from build123d import *

# Parameters (mm, degrees)
SALIENTE_EXTRUIR1_OUTLINE_R = 1.5
SALIENTE_EXTRUIR1_DEPTH     = 3
S_LIDO_MOVER_COPIAR1_ANGLE  = 90


# Read off the part's stored shape, not the designer's step: Saliente-Extruir1
with BuildPart() as part:
    # Saliente-Extruir1 outline → Saliente-Extruir1 (new body)
    with BuildSketch(Plane.XY):
        with BuildLine():
            ThreePointArc((41771.487432324, -438.916733549), (41774.992492467, -434.200692189), (41770.014438295, -431.078918755))
            ThreePointArc((41770.014438295, -431.078918755), (41751.456517689, -433.102313751), (41733.174949659, -429.324111148))
            ThreePointArc((41733.174949659, -429.324111148), (41725.991842174, -431.730062122), (41726.889701646, -439.251995491))
            ThreePointArc((41726.889701646, -439.251995491), (41729.909074744, -445.69247761), (41727.882942515, -452.510924062))
            ThreePointArc((41727.882942515, -452.510924062), (41728.480324995, -457.995391332), (41733.987432324, -457.666733549))
            ThreePointArc((41733.987432324, -457.666733549), (41751.046402032, -444.909672965), (41771.487432324, -438.916733549))
        make_face()
        with Locations((41731.061313295, -454.939495491)):
            Circle(SALIENTE_EXTRUIR1_OUTLINE_R, mode=Mode.SUBTRACT)
        with BuildLine():
            Line((41738.411012413, -442.993278413), (41736.838856305, -443.404992792))
            ThreePointArc((41736.838856305, -443.404992792), (41735.982036246, -443.234989406), (41735.585699802, -442.456555601))
            ThreePointArc((41735.585699802, -442.456555601), (41735.69345686, -441.876829753), (41736.169165633, -441.52841218))
            Line((41736.169165633, -441.52841218), (41737.831630416, -441.093055392))
            ThreePointArc((41737.831630416, -441.093055392), (41738.100055673, -441.068468468), (41738.361410126, -441.134426674))
            Line((41738.361410126, -441.134426674), (41742.678233483, -443.044025097))
            Line((41742.678233483, -443.044025097), (41742.08574273, -437.173422628))
            ThreePointArc((41742.08574273, -437.173422628), (41742.914855043, -435.985031701), (41744.060436871, -436.872354922))
            Line((41744.060436871, -436.872354922), (41744.754133415, -443.73758562))
            ThreePointArc((41744.754133415, -443.73758562), (41744.580022463, -444.529990261), (41743.875600122, -444.932493559))
            Line((41743.875600122, -444.932493559), (41742.980225481, -445.023621226))
            Line((41742.980225481, -445.023621226), (41738.411012413, -442.993278413))
        make_face(mode=Mode.SUBTRACT)
        with Locations((41731.061313295, -434.939495491)):
            Circle(SALIENTE_EXTRUIR1_OUTLINE_R, mode=Mode.SUBTRACT)
        with Locations((41771.061313295, -434.939495491)):
            Circle(SALIENTE_EXTRUIR1_OUTLINE_R, mode=Mode.SUBTRACT)
    extrude(amount=SALIENTE_EXTRUIR1_DEPTH)


with BuildPart() as part_1:
    # Sólido-Mover/Copiar1: moved
    add(part.part.rotate(Axis((0, -443.939495491, 1.5), (-1, 0, 0)), S_LIDO_MOVER_COPIAR1_ANGLE))


solid = part_1.part
Here's how the part is built. I have some questions about the finished solid (model axes, mm). A direction names the side the tool comes from. Give positions to 0.01 mm unless a question says otherwise; leave off trailing zeros. Loops run counter-clockwise (first coordinate to the right, second up) from the corner with the lowest first, then second, coordinate; pieces in that order, holes last. Notation, with made-up numbers: (-18, 78) -> (19, 78) arc R37 ccw to (19, 114) -> close; hole circle Ø3 at (26, -0.75). An arc over 180 degrees is marked (long way). Answer as a JSON object with one key per item and string values. Group by question number.
Item 1: Thinking about a two-plate mould opening in Z: for faces 3 (the flat face through (41739, -442.439, -2)), 4 (the cylindrical face through (41750.779, -443.96, 2.605)), 5 (the cylindrical face through (41728.416, -443.96, 15.5)), which applies, pulls with the +Z half, pulls with the -Z half, needs draft (parallel to the pull), parting line crosses it, or undercut?
Item 2: Will these pins go through, and if not, where does the flat tip stop? pin 1 (2.5 mm diameter, centred on x = 41731.06, z = 12.5, fed in from +Y); pin 2 (4 mm diameter, centred on x = 41731.06, z = -7.5, fed in from -Y); pin 3 (1 mm diameter, centred on y = -445, z = 7.5, fed in from +X).
Item 3: Imagine slicing it at A-A on z = -7.5. Write out the boundary of the cut face in (x, y).
Item 4: I need wall thicknesses on L1, parallel to X at y = -443.25, z = -7.5; L2, parallel to Z at x = 41730.5, y = -444.05; L3, parallel to X at y = -443.6, z = -5. Which ranges of each line are inside material? Lowest first, please.
Item 5: On a 3-axis mill with a long thin cutter (end or side, diameter ignored), from which of +Z, -Z, +X, -X, +Y, -Y can I reach the whole of each face in a straight line? I mean faces 1 (the flat face through (41736.989, -443.96, -1.126)), 2 (the cylindrical face through (41751.719, -443.96, -9.325)). Say none if no direction works.
Item 6: Imagine slicing it at D-D on z = 12.5. Write out the boundary of the cut face in (x, y), then the cut area to 3 significant figures.
Item 7: Imagine slicing it at B-B on y = -443.7. Write out the boundary of the cut face in (x, z), then the cut area to 3 significant figures.
Item 8: Imagine slicing it at C-C on x = 41772. Write out the boundary of the cut face in (y, z).
Answer list:
{
 "1": {"face 3": "needs draft", "face 4": "pulls with the +Z half", "face 5": "undercut"},
 "2": {"pin 1": "passes through", "pin 2": "stops at y = -445.44", "pin 3": "stops at x = 41743.45"},
 "3": {"outline": "(41725.06, -445.44) -> (41729.56, -445.44) -> (41729.56, -442.44) -> (41725.06, -442.44) -> close; (41732.56, -445.44) -> (41769.56, -445.44) -> (41769.56, -442.44) -> (41732.56, -442.44) -> close; (41772.56, -445.44) -> (41775.06, -445.44) -> (41775.06, -442.44) -> (41772.56, -442.44) -> close"},
 "4": {"L1": "x = 41725.06 to 41729.56, 41732.56 to 41769.56, 41772.56 to 41775.06", "L2": "z = -13.47 to -8.89, -6.11 to 11.11, 13.89 to 16.46", "L3": "x = 41725.61 to 41742.11, 41744.12 to 41774.18"},
 "5": {"face 1": "+Y, -Y", "face 2": "-Z, +Y, -Y"},
 "6": {"outline": "(41727.06, -445.44) -> (41729.56, -445.44) -> (41729.56, -442.44) -> (41727.06, -442.44) -> close; (41732.56, -445.44) -> (41736.7, -445.44) -> (41736.7, -442.44) -> (41732.56, -442.44) -> close", "area": "19.9 mm2"},
 "7": {"outline": "(41726.89, -3.19) arc R6 ccw to (41733.17, -13.12) arc R60 cw to (41770.01, -11.36) arc R4 ccw (long way) to (41771.49, -3.52) arc R60 cw to (41733.99, 15.23) arc R4 ccw to (41727.88, 10.07) arc R10 cw to start; hole circle Ø3 at (41731.06, -7.5); hole circle Ø3 at (41731.06, 12.5); hole (41735.59, 0.02) arc R0.8 ccw to (41736.17, -0.91) -> (41737.83, -1.35) arc R0.8 ccw to (41738.36, -1.31) -> (41742.68, 0.6) -> (41742.09, -5.27) arc R1 ccw (long way) to (41744.06, -5.57) -> (41744.75, 1.3) arc R1 ccw to (41743.88, 2.49) -> (41742.98, 2.58) -> (41738.41, 0.55) -> (41736.84, 0.97) arc R1 ccw to start; hole circle Ø3 at (41771.06, -7.5)", "area": "653 mm2"},
 "8": {"outline": "(-445.44, -11.39) -> (-442.44, -11.39) -> (-442.44, -8.67) -> (-445.44, -8.67) -> close; (-445.44, -6.33) -> (-442.44, -6.33) -> (-442.44, -3.61) -> (-445.44, -3.61) -> close"}
}
